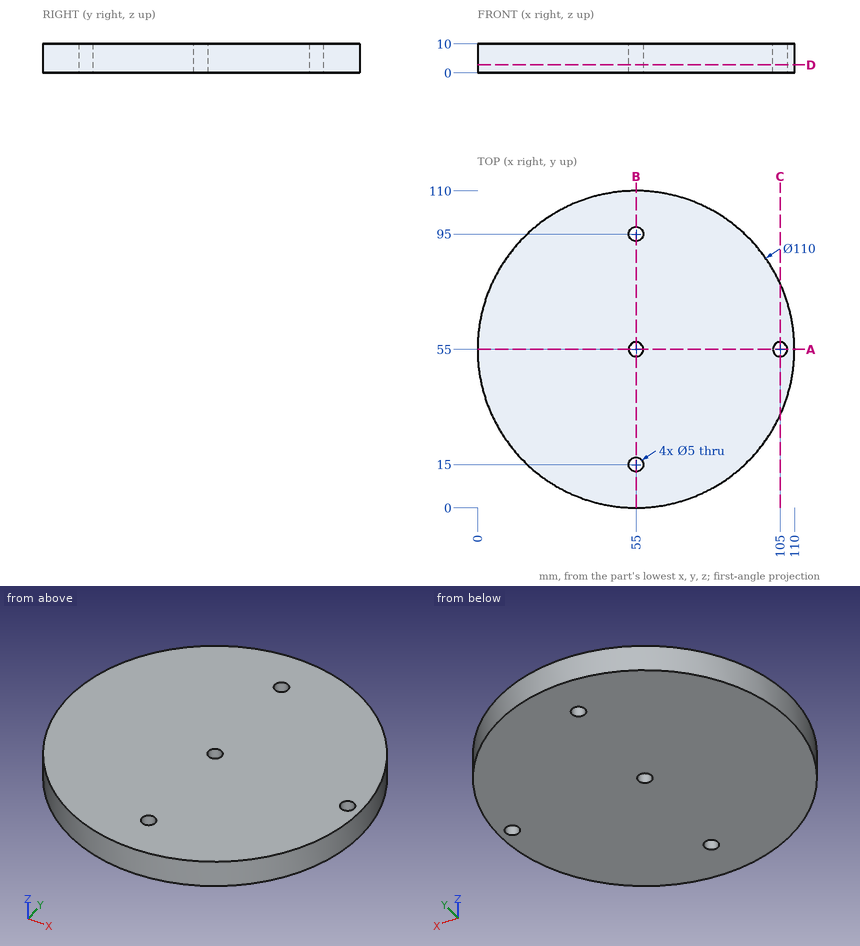
Can you work these out from the drawing? Everything is in mm from the part's minimum corner. Round coordinates to 2 decimals unless told otherwise and drop trailing zeros. Loops run counter-clockwise (first coordinate to the right, second up) from the corner with the lowest first, then second, coordinate; pieces in that order, holes last. Notation, with made-up numbers: M 21,0 L 71,0 A21 ccw 71,35 Z; hole C 24,88 d6. An arc over 180 degrees is marked long. Write item = value, one per line.
1. I need wall thicknesses on probe 1 along Y at (x, z) = (55, 2.5); probe 2 along Y at (x, z) = (105, 2); probe 3 along X at (y, z) = (95, 5.75). Which ranges of each line are inside material? Lowest first, please.
Results below:
probe_1 = 0 to 12.5, 17.5 to 52.5, 57.5 to 92.5, 97.5 to 110
probe_2 = 32.09 to 52.5, 57.5 to 77.91
probe_3 = 17.25 to 52.5, 57.5 to 92.75
2. I want a section at D-D, the plane z = 2.75. Write out the boundary of the cut face in (x, y).
Results below:
outline = C 55,55 d110; hole C 55,15 d5; hole C 55,55 d5; hole C 55,95 d5; hole C 105,55 d5
3. I want a section at A-A, the plane y = 55. Write out the boundary of the cut face in (x, z).
Results below:
outline = M 0,0 L 52.5,0 L 52.5,10 L 0,10 Z; M 57.5,0 L 102.5,0 L 102.5,10 L 57.5,10 Z; M 107.5,0 L 110,0 L 110,10 L 107.5,10 Z
4. I want a section at B-B, the plane x = 55. Write out the boundary of the cut face in (y, z).
Results below:
outline = M 0,0 L 12.5,0 L 12.5,10 L 0,10 Z; M 17.5,0 L 52.5,0 L 52.5,10 L 17.5,10 Z; M 57.5,0 L 92.5,0 L 92.5,10 L 57.5,10 Z; M 97.5,0 L 110,0 L 110,10 L 97.5,10 Z
5. Will these pins go through, and if not, where does the flat tip stop? P1, Ø1.5, axis at x = 34, z = 4, coming from the +Y side; P2, Ø4.5, axis at x = 55, y = 55, coming from the +Z side; P3, Ø5, axis at x = 12.5, z = 1.5, coming from the -Y side; P4, Ø6, axis at x = 79, z = 5, coming from the -Y side.
Results below:
P1 = 106.14
P2 = through
P3 = 17.25
P4 = 4.17
6. I want a section at C-C, the plane x = 105. Write out the boundary of the cut face in (y, z).
Results below:
outline = M 32.09,0 L 52.5,0 L 52.5,10 L 32.09,10 Z; M 57.5,0 L 77.91,0 L 77.91,10 L 57.5,10 Z
